For this review, take the finished solid that the model builds, in its own axes (mm). Face numbers are marked on the shaded views. A direction names the side the tool comes from. Round coordinates to 2 decimals unless told otherwise and drop trailing zeros. Write each loop counter-clockwise with the first axis right and the second up, starting at its lowest first coordinate (ties: lowest second). Pieces come first, ordered by that corner, then holes. Notation, with made-up numbers: (44.5, 81) - (73.5, 81) arc R17 cw to (73.5, 111) - close; hole circle Ø4 at (-12.5, -20). An arc over 180 degrees is marked (long way). Answer in a Markdown table with one row per item. Add a question column.
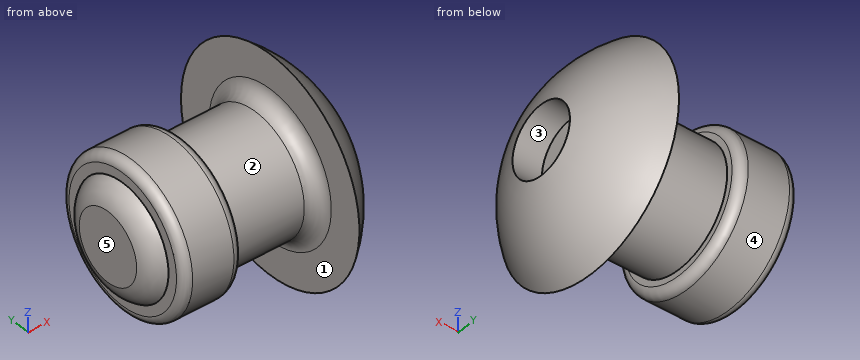
from build123d import *

# Parameters (mm, degrees)
FILLET1_R      = 0.5
CHAMFER1_SIZE  = 2.35
CHAMFER1_SIZE2 = 0.629680602
SKETCH_1_W     = 29
SKETCH_1_H     = 1.175


with BuildPart() as part:
    # Sketch1 → Base-Revolve (revolve)
    with BuildSketch(Plane(origin=(-11.603452862, 14.723452862, 0), x_dir=(0, -1, 0), z_dir=(0, 0, 1)), mode=Mode.PRIVATE) as base_revolve_sk:
        with BuildLine():
            Line((16.923452862, 12.103452862), (16.598206218, 12.103452862))
            ThreePointArc((16.598206218, 12.103452862), (16.304826689, 11.774384722), (15.898452862, 11.603452862))
            Line((15.898452862, 11.603452862), (14.723452862, 11.603452862))
            Line((14.723452862, 11.603452862), (14.723452862, 46.750877613))
            Line((14.723452862, 46.750877613), (15.898452862, 46.750877613))
            Line((15.898452862, 46.750877613), (15.898452862, 18.750877613))
            ThreePointArc((15.898452862, 18.750877613), (17.272699482, 18.132605809), (18.373452862, 17.103452862))
            Line((18.373452862, 17.103452862), (16.723452862, 17.103452862))
            Line((16.723452862, 17.103452862), (16.723452862, 14.103452862))
            Line((16.723452862, 14.103452862), (16.923452862, 14.103452862))
            ThreePointArc((16.923452862, 14.103452862), (17.135584897, 14.015584897), (17.223452862, 13.803452862))
            Line((17.223452862, 13.803452862), (17.223452862, 12.403452862))
            ThreePointArc((17.223452862, 12.403452862), (17.135584897, 12.191320828), (16.923452862, 12.103452862))
        make_face()
    revolve(base_revolve_sk.sketch.rotate(Axis((22.234231882, 0, 0), (-1, 0, 0)), 180), axis=Axis((22.234231882, 0, 0), (-1, 0, 0)))

    # Fillet1
    fillet1_edges = [part.edges().sort_by_distance(p)[0] for p in [
        (5.5, -2, 0),
    ]]
    fillet(fillet1_edges, radius=FILLET1_R)

    # Chamfer1
    chamfer1_edges = [part.edges().sort_by_distance(p)[0] for p in [
        (35.14742475, -1.175, 0),
    ]]
    chamfer1_side = [part.faces().sort_by_distance(p)[0] for p in [
        (21.14742475, -1.175, 0),
    ]]
    chamfer(chamfer1_edges, length=CHAMFER1_SIZE, length2=CHAMFER1_SIZE2, reference=chamfer1_side[0])

    # Эскиз1 → Вырез-Повернуть1 (revolve, cut)
    with BuildSketch(Plane(origin=(0, 0, 0), x_dir=(1, 0, 0), z_dir=(0, 1, 0))):
        with Locations((20.64742475, 0.5875)):
            Rectangle(SKETCH_1_W, SKETCH_1_H)
    revolve(axis=Axis((35.14742475, 0, 0), (-1, 0, 0)), mode=Mode.SUBTRACT)


solid = part.part
Q1. To check wall thickness, follow probe 1 along X at (y, z) = (2, 1); probe 2 along Z at (x, y) = (6.6, 0) (3 decimals); probe 3 along X at (y, z) = (2.25, 0.75). State the ranges of each line that lie inside material, in increasing order.
Q2. Insertion check: pin 1 Ø1.5 at (y, z) = (1.5, 1.5) entering from +X; pin 2 Ø2 at (y, z) = (-0.5, 0.5) entering from -X; pin 3 Ø2 at (y, z) = (0, 0) entering from +X; pin 4 Ø1.5 at (x, y) = (5.5, 1.5) entering from -Z. Each pin has a flat end and moves straight along its axis. Give the tip position at first contact, or say it passes through.
Q3. Draft analysis for pull direction Y (two halves, no side actions). For the marked faces 1, 2 and 3, state which applies: released by +Y, released by -Y, zero draft, split by the parting line, or undercut.
Q4. Tool access review of the marked faces 4 and 5: name each direction out of +Z, -Z, +X, -X, +Y, -Y from which nothing blocks a thin tool from reaching the whole face with its end or side.
Q5. Add section A-A on y = 0. State the section outline as (x, z) points (3 decimals).
Q6. Add section D-D on z = -3. State the section outline as (x, y) points, then the cut area to 3 significant figures.
Q7. Add section C-C on x = 3.75. State the section outline as (y, z) points, then the cut area to 3 significant figures.
Answer sheet:
| question | item | result |
|---|---|---|
| 1 | probe 1 | x = 0.5 to 2.5, 5.42 to 6.72 |
| 1 | probe 2 | z = -2.439 to -1.175, 1.175 to 2.439 |
| 1 | probe 3 | x = 0.55 to 2.45, 5.48 to 6.64 |
| 2 | pin 1 | stops at x = 7.09 |
| 2 | pin 2 | stops at x = 0 |
| 2 | pin 3 | stops at x = 6.15 |
| 2 | pin 4 | stops at z = -3.57 |
| 3 | face 1 | zero draft |
| 3 | face 2 | split by the parting line |
| 3 | face 3 | undercut |
| 4 | face 4 | -X |
| 4 | face 5 | +Z, -Z, -X, +Y, -Y |
| 5 | outline | (0, -1.175) arc R1 ccw to (0.5, -1.875) - (0.5, -2.2) arc R0.3 ccw to (0.8, -2.5) - (2.2, -2.5) arc R0.3 ccw to (2.5, -2.2) - (2.5, -2) - (5, -2) arc R0.5 cw to (5.5, -2.5) - (5.5, -3.65) arc R4.601 ccw to (7.147, -1.175) - (6.147, -1.175) - (6.147, 1.175) - (7.147, 1.175) arc R4.601 ccw to (5.5, 3.65) - (5.5, 2.5) arc R0.5 cw to (5, 2) - (2.5, 2) - (2.5, 2.2) arc R0.3 ccw to (2.2, 2.5) - (0.8, 2.5) arc R0.3 ccw to (0.5, 2.2) - (0.5, 1.875) arc R1 ccw to (0, 1.175) - close |
| 6 | outline | (5.5, -2.08) arc R3.49 ccw to (5.5, 2.08) - close |
| 6 | area | 1.95 mm² |
| 7 | outline | circle Ø4 at (0, 0) |
| 7 | area | 12.6 mm² |
